Could you check a few things on this model? Use its own coordinates, in mm. A direction names the side the tool comes from. Give positions to 0.01 mm unless a question says otherwise; leave off trailing zeros. Order: outer loops, then holes, each group sorted by start corner. A loop starts at its lowest first (then second) coordinate and runs counter-clockwise, first axis right, second up.
from build123d import *

# Parameters (mm, degrees)
F1_DEPTH = 100
F2_R     = 2.25
F3_DEPTH = 5
F4_DEPTH = 25


with BuildPart() as f1:
    # F0 (on Front) → F1 (new body)
    with BuildSketch(Plane.XZ):
        with BuildLine():
            ThreePointArc((10.9544511501, 1), (0, 11), (-10.9544511501, 1))
            Line((-10.9544511501, 1), (10.9544511501, 1))
        make_face()
    extrude(amount=F1_DEPTH)

    # F2 (on face) → F3 (cut)
    with BuildSketch(Plane(origin=(0, 0, 1), x_dir=(1, 0, 0), z_dir=(0, 0, -1))):
        Polygon((-2.0784609691, 2.65), (2.0784609691, 2.65), (4.1569219382, 6.25), (2.0784609691, 9.85), (-2.0784609691, 9.85), (-4.1569219382, 6.25), align=None)
        with Locations((0, 6.25)):
            Circle(F2_R, mode=Mode.SUBTRACT)
        Polygon((-2.0784609691, 78.9), (2.0784609691, 78.9), (4.1569219382, 82.5), (2.0784609691, 86.1), (-2.0784609691, 86.1), (-4.1569219382, 82.5), align=None)
        with Locations((0, 82.5)):
            Circle(F2_R, mode=Mode.SUBTRACT)
    extrude(amount=-F3_DEPTH, mode=Mode.SUBTRACT)

    # F4 (cut): faces of the model
    f4_faces = [f1.faces().sort_by_distance(p)[0] for p in [
        (0, -82.5, 1),
        (0, -6.25, 1),
    ]]
    extrude(f4_faces, amount=-F4_DEPTH, mode=Mode.SUBTRACT)


solid = f1.part
Item 1: We'd pull the mould along Y, two halves only. Please class faces 1 (the flat face through (0, -49, 1)), 2 (the flat face through (0, -100, 5)), 3 (the flat face through (0, -78.9, 3)), 4 (the flat face through (3.1, -80.67, 3.46)): +Y half, -Y half, draft (parallel to the pull), parting line (faces both ways), or undercut.
Findings:
face 1: draft
face 2: -Y half
face 3: undercut
face 4: undercut
Item 2: For faces 5 (the cylindrical face through (-0.488, -80.304, 8.468)), 6 (the flat face through (-3.1, -8.08, 3.46)), which set-ups out of +Z, -Z, +X, -X, +Y, -Y let a thin tool reach every point of the face, with its end or its side?
Findings:
face 5: +Z, -Z
face 6: -Z
Item 3: Imagine slicing it at B-B on z = 2.5. List the corners of the cut face in (x, y) for me, then the cut area to 3 significant figures.
Findings:
outline: (-10.71, -100) - (10.71, -100) - (10.71, 0) - (-10.71, 0) - close; hole (-4.16, -82.5) - (-2.08, -86.1) - (2.08, -86.1) - (4.16, -82.5) - (2.08, -78.9) - (-2.08, -78.9) - close; hole (-4.16, -6.25) - (-2.08, -9.85) - (2.08, -9.85) - (4.16, -6.25) - (2.08, -2.65) - (-2.08, -2.65) - close
area: 2,050 mm2
Item 4: Please list where these lines run through material, in increasing order: line 1 along Y through (x, z) = (0, 8.6); line 2 along Y through (x, z) = (-0.5, 4.75); line 3 along X through (y, z) = (-6.25, 7.8).
Findings:
line 1: y = -100 to -84.75, -80.25 to -8.5, -4 to 0
line 2: y = -100 to -86.1, -78.9 to -9.85, -2.65 to 0
line 3: x = -7.76 to -2.25, 2.25 to 7.76
Item 5: For pin 1 (6 mm diameter, centred on x = 7.5, y = -61.5, fed in from +Z), with a flat end and sliding along its axis, tell me the tip position at first contact or that it passes through.
Findings:
pin 1: stops at z = 10.04
Item 6: Imagine slicing it at C-C on y = -53. List the corners of the cut face in (x, z) for me.
Findings:
outline: (-10.95, 1) - (10.95, 1) arc R11 ccw to start
Item 7: Imagine slicing it at D-D on z = 7.25. List the corners of the cut face in (x, y) for me, then the cut area to 3 significant figures.
Findings:
outline: (-8.27, -100) - (8.27, -100) - (8.27, 0) - (-8.27, 0) - close; hole circle Ø4.5 at (0, -82.5); hole circle Ø4.5 at (0, -6.25)
area: 1,620 mm2
Item 8: Imagine slicing it at A-A on x = 0. List the corners of the cut face in (y, z) for me.
Findings:
outline: (-100, 1) - (-86.1, 1) - (-86.1, 6) - (-84.75, 6) - (-84.75, 11) - (-100, 11) - close; (-80.25, 6) - (-78.9, 6) - (-78.9, 1) - (-9.85, 1) - (-9.85, 6) - (-8.5, 6) - (-8.5, 11) - (-80.25, 11) - close; (-4, 6) - (-2.65, 6) - (-2.65, 1) - (0, 1) - (0, 11) - (-4, 11) - close
